Check sheet for the modelled part. Datum: model origin and axes. Units: mm. A direction names the side the tool comes from. Round coordinates to 2 decimals unless told otherwise and drop trailing zeros. Order: outer loops, then holes, each group sorted by start corner. A loop starts at its lowest first (then second) coordinate and runs counter-clockwise, first axis right, second up.
(1) Sectioned sample at C-C, the plane z = -2.75. Enter the section's corners in (x, y) (1 decimal).
(2) Thickness scan on probe 1 along Z at (x, y) = (-12.7, -7.05); probe 2 along Y at (x, z) = (56, 1.25); probe 3 along Y at (x, z) = (40, -3.5). Record the ranges inside material, lowest first.
(3) Depth check by flat-ended pin: pin 1 (2.5 mm diameter, centred on x = -12.7, z = 3.47, fed in from -Y); pin 2 (5.5 mm diameter, centred on x = 63.5, z = -6.05, fed in from +Y); pin 3 (5.5 mm diameter, centred on x = 27, y = 2, fed in from +Z); pin 4 (6 mm diameter, centred on x = 40.5, z = -3.5, fed in from +Y). Enter the tip coordinate at first touch or a pass-through.
(4) Tool access check on faces 4 (the cylindrical face through (25.76, -5.16, 3.7)), 5 (the cylindrical face through (-11, -6.8, 3.4)). Record the directions out of +Z, -Z, +X, -X, +Y, -Y that give a thin tool (end or side, any length) a straight path to the whole face; none if there is none.
(5) Sectioned sample at B-B, the plane y = -3. Enter the section's corners in (x, z), and give its area (3 significant figures).
(6) Sectioned sample at D-D, the plane y = 2.5. Enter the section's corners in (x, z), and give its area (3 significant figures).
(7) Mould release check, pull along X, two halves, no side actions. Record for faces 1 (the flat face through (25, -6.033, 0)), 2 (the flat face through (25.5, 4.2, 5.04)), 3 (the flat face through (-15.875, -7, -1)): released by +X, released by -X, zero draft, split by the parting line, or undercut.
```python
from build123d import *

# Parameters (mm, degrees)
SKETCH2_W            = 5.08
SKETCH2_H            = 11.43
CUT_EXTRUDE1_DEPTH   = 76.2
SKETCH3_W            = 82.55
SKETCH3_H            = 15.875
BOSS_EXTRUDE1_DEPTH  = 1.5875
M3_CLEARANCE_HOLE1_D = 3.4


# Read off the part's stored shape, not the designer's step: Shell1
with BuildPart() as part:
    # Sketch1 → Revolve1 (revolve)
    with BuildSketch(Plane.XY):
        with BuildLine():
            Line((0, 7.62), (50.8, 7.62))
            ThreePointArc((50.8, 7.62), (56.188153673, 5.388153673), (58.42, 0))
            Line((58.42, 0), (-7.62, 0))
            ThreePointArc((-7.62, 0), (-5.388153673, 5.388153673), (0, 7.62))
        make_face()
    revolve(axis=Axis((0, 0, 0), (1, 0, 0)))

    # Sketch2 → Cut-Extrude1 (cut, symmetric)
    with BuildSketch(Plane(origin=(0, 0, 0), x_dir=(0, 0, -1), z_dir=(1, 0, 0))):
        with Locations((-7.580156248, 0)):
            Rectangle(SKETCH2_W, SKETCH2_H)
    extrude(amount=CUT_EXTRUDE1_DEPTH, both=True, mode=Mode.SUBTRACT)

    # Shell1 outline → Shell1 (revolve, cut)
    with BuildSketch(Plane.YX):
        with BuildLine():
            Line((0, 57.15), (0, -6.35))
            ThreePointArc((0, -6.35), (4.490128063, -4.490128058), (6.35, 6e-09))
            Line((6.35, 6e-09), (6.35, 50.799999994))
            ThreePointArc((6.35, 50.799999994), (4.490128063, 55.290128058), (0, 57.15))
        make_face()
    revolve(axis=Axis((0, 0, 0), (1, 0, 0)), mode=Mode.SUBTRACT)

    # Sketch3 → Boss-Extrude1 (add)
    with BuildSketch(Plane(origin=(0, -7.62, 0), x_dir=(1, 0, 0), z_dir=(0, 1, 0))):
        with Locations((25.4, 1.289921876)):
            Rectangle(SKETCH3_W, SKETCH3_H)
    extrude(amount=BOSS_EXTRUDE1_DEPTH)

    # M3 Clearance Hole1 (through all)
    with Locations(Plane(origin=(0, -6.0325, 0), x_dir=(1, 0, 0), z_dir=(0, 1, 0))):
        with Locations((-12.7, 6.052421876), (-12.7, -3.472578124), (63.5, 6.052421876), (63.5, -2.26916829)):
            Hole(M3_CLEARANCE_HOLE1_D / 2)


solid = part.part
```
Derived:
1. outline: (-15.9, -7.6) - (66.7, -7.6) - (66.7, -6) - (54.6, -6) arc R7.1 ccw to (50.8, 7.1) - (0, 7.1) arc R7.1 ccw to (-3.8, -6) - (-15.9, -6) - close; hole (0, -5.7) - (50.8, -5.7) arc R5.7 ccw to (50.8, 5.7) - (0, 5.7) arc R5.7 ccw to start
2. probe 1: z = -9.23 to -7.75, -4.35 to 1.77, 5.17 to 6.65
2. probe 2: y = -7.62 to -6.03, -5.43 to -3.42, 3.42 to 5.43
2. probe 3: y = -7.62 to -5.3, 5.3 to 6.77
3. pin 1: passes through
3. pin 2: stops at y = -6.03
3. pin 3: stops at z = 5.04
3. pin 4: stops at y = 7.6
4. face 4: none
4. face 5: +Y, -Y
5. outline: (-4.86, 5.04) arc R7 ccw to (0, -7) - (50.8, -7) arc R7 ccw to (55.66, 5.04) - (53.23, 5.04) arc R5.6 cw to (50.8, -5.6) - (0, -5.6) arc R5.6 cw to (-2.43, 5.04) - close
5. area: 116 mm2
6. outline: (-5.14, 5.04) arc R7.2 ccw to (0, -7.2) - (50.8, -7.2) arc R7.2 ccw to (55.94, 5.04) - (53.74, 5.04) arc R5.84 cw to (50.8, -5.84) - (0, -5.84) arc R5.84 cw to (-2.94, 5.04) - close
6. area: 113 mm2
7. face 1: undercut
7. face 2: zero draft
7. face 3: released by -X
